Study the drawing (mm; zero at the part's minimum x, y, z) and answer. A direction names the side the tool comes from. Coordinates: 2 decimals unless noted, no trailing zeros. Order: outer loops, then holes, each group sorted by start corner. A loop starts at its lowest first (then second) coordinate and runs counter-clockwise, first axis right, second up.
1. Determine the mould class of the marked faces 1, 2, 3 and 4 for opening direction Z: +Z half, -Z half, draft (parallel to the pull), parting line (faces both ways), or undercut.
2. Flat-ended cylindrical pins translate along their axes: pin 1 Ø4 at (x, y) = (34, 6) entering from +Z; pin 2 Ø7 at (y, z) = (9.5, 19) entering from -X; pin 3 Ø2 at (y, z) = (7, 27.5) entering from +X. Find the tip coordinate at first contact, or state that the pin passes through.
3. The part is cut by section A-A, the plane z = 20. Give the vertices of the cut face in (x, y).
4. Find the intervals of material crossed by probe 1 along Y at (x, z) = (5, 3.35); probe 2 along Z at (x, y) = (21, 10.75); probe 3 along X at (y, z) = (10.25, 26), in increasing order.
5. A tool of negligible diameter and unlimited length cuts with its end or side. For the marked faces 5, 6 and 7, from which of +Z, -Z, +X, -X, +Y, -Y can it reach the whole face along a straight path? Write none if from no direction.
6. The part is cut by section C-C, the plane y = 2. Give the vertices of the cut face in (x, z).
7. The part is cut by section D-D, the plane z = 25. Give the vertices of the cut face in (x, y), then the cut area to 3 significant figures.
8. The part is cut by section B-B, the plane x = 37. Give the vertices of the cut face in (y, z).
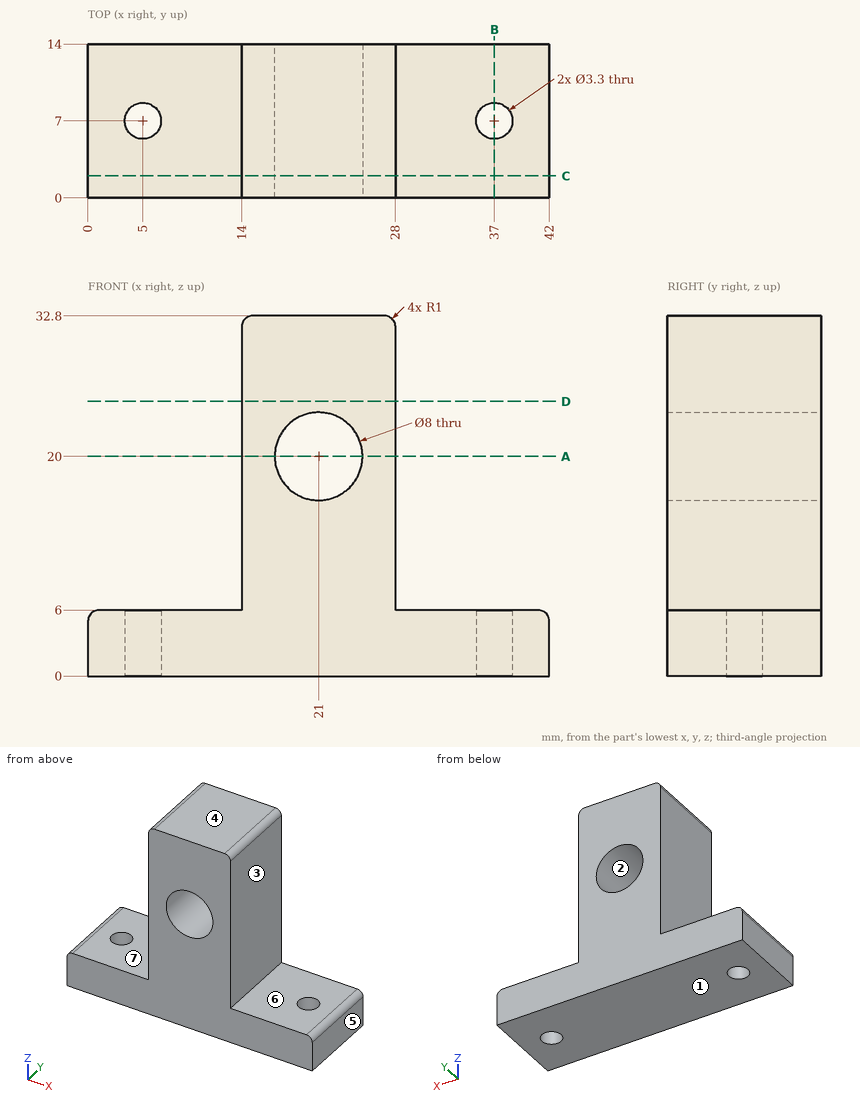
Geometry says:
1. face 1: -Z half
1. face 2: undercut
1. face 3: draft
1. face 4: +Z half
2. pin 1: stops at z = 6
2. pin 2: stops at x = 14
2. pin 3: stops at x = 28
3. outline: (14, 0) - (17, 0) - (17, 14) - (14, 14) - close; (25, 0) - (28, 0) - (28, 14) - (25, 14) - close
4. probe 1: y = 0 to 5.35, 8.65 to 14
4. probe 2: z = 0 to 16, 24 to 32.8
4. probe 3: x = 14 to 28
5. face 5: +Z, -Z, +X, +Y, -Y
5. face 6: +Z, +X, +Y, -Y
5. face 7: +Z, -X, +Y, -Y
6. outline: (0, 0) - (42, 0) - (42, 5) arc R1 ccw to (41, 6) - (28, 6) - (28, 31.8) arc R1 ccw to (27, 32.8) - (15, 32.8) arc R1 ccw to (14, 31.8) - (14, 6) - (1, 6) arc R1 ccw to (0, 5) - close; hole circle Ø8 at (21, 20)
7. outline: (14, 0) - (28, 0) - (28, 14) - (14, 14) - close
7. area: 196 mm2
8. outline: (0, 0) - (5.35, 0) - (5.35, 6) - (0, 6) - close; (8.65, 0) - (14, 0) - (14, 6) - (8.65, 6) - close
